Read the model definition and answer for the solid it produces. Units are mm, in the model's axes. A direction names the side the tool comes from. Coordinates: 2 decimals unless noted, no trailing zeros. Order: outer loops, then holes, each group sorted by start corner. A loop starts at its lowest first (then second) coordinate and runs counter-clockwise, first axis right, second up. Notation, with made-up numbers: (14, 3.25) -> (19, 3.25) arc R12 ccw to (19, 19.25) -> close; hole circle Ø4 at (64, 66.5). An arc over 180 degrees is marked (long way). Use CSV: the item, a comma, the result in double quotes.
```python
from build123d import *

# Parameters (mm, degrees)
F1_DEPTH = 7.14375
F2_W     = 15.875
F2_H     = 14.2875
F3_DEPTH = 9.525


with BuildPart() as f1:
    # F0 (on Top) → F1 (new body, symmetric)
    with BuildSketch(Plane.XY):
        Polygon((40.48125, 53.975), (40.48125, 9.525), (-40.48125, 9.525), (-40.48125, 53.975), (-53.18125, 53.975), (-53.18125, 9.525), (-53.18125, -9.525), (-40.48125, -9.525), (40.48125, -9.525), (53.18125, -9.525), (53.18125, 9.525), (53.18125, 53.975), align=None)
    extrude(amount=F1_DEPTH, both=True)

    # F2 (on face) → F3 (join)
    with BuildSketch(Plane(origin=(-53.18125, 0, 0), x_dir=(0, -1, 0), z_dir=(-1, 0, 0))):
        with Locations((-38.1, 0)):
            Rectangle(F2_W, F2_H)
    extrude(amount=F3_DEPTH)


solid = f1.part
```
Item 1: Find section A-A, the plane y = 19. Give the vertices of the cut face in (x, z).
Return value:
outline,"(-53.18, -7.14) -> (-40.48, -7.14) -> (-40.48, 7.14) -> (-53.18, 7.14) -> close; (40.48, -7.14) -> (53.18, -7.14) -> (53.18, 7.14) -> (40.48, 7.14) -> close"
Item 2: Straight lines are drawn through the part: line 1 along X through (y, z) = (43.5, -2.25); line 2 along X through (y, z) = (12.5, 1.25); line 3 along X through (y, z) = (-6.5, 0.75). For each, find the intervals that lie inside material, in ascending order.
Return value:
line 1,"x = -62.71 to -40.48, 40.48 to 53.18"
line 2,"x = -53.18 to -40.48, 40.48 to 53.18"
line 3,"x = -53.18 to 53.18"
Item 3: The mould has two halves that part along X. Classify faces 1 (the flat face through (-6, 9, -7.144)), 2 (the flat face through (1, 9.525, 0)), 3 (the flat face through (-40.481, 31, 0)), 4 (the flat face through (53.181, 22, 0)): +X half, -X half, draft (parallel to the pull), parting line (faces both ways), or undercut.
Return value:
face 1,"draft"
face 2,"undercut"
face 3,"undercut"
face 4,"+X half"
Item 4: A tool of negligible diameter and unlimited length cuts with its end or side. For faces 5 (the flat face through (-58, 30.162, 0)), 6 (the flat face through (40.481, 32, 0)), 7 (the flat face through (-6, 9, 7.144)), 8 (the flat face through (-53.181, 50, 0)), from which of +Z, -Z, +X, -X, +Y, -Y can it reach the whole face along a straight path? Write none if from no direction.
Return value:
face 5,"+Z, -Z, -X, -Y"
face 6,"+Z, -Z, +Y"
face 7,"+Z, +X, -X, +Y, -Y"
face 8,"+Z, -Z, -X, +Y"
Item 5: Find section C-C, the plane y = 33.5. Give the vertices of the cut face in (x, z).
Return value:
outline,"(-62.71, -7.14) -> (-40.48, -7.14) -> (-40.48, 7.14) -> (-62.71, 7.14) -> close; (40.48, -7.14) -> (53.18, -7.14) -> (53.18, 7.14) -> (40.48, 7.14) -> close"
Item 6: Each of these flat-tipped pins is pushed along its axis until it touches: P1, Ø4, axis at y = 6.5, z = 3.5, coming from the -X side; P2, Ø7.5, axis at x = -57, z = 1, coming from the +Y side; P3, Ø4.5, axis at x = -0.5, z = -1, coming from the +Y side (3 decimals). Where does it stop, or does it pass through?
Return value:
P1,"stops at x = -53.18"
P2,"stops at y = 46.04"
P3,"stops at y = 9.525"
Item 7: Find section B-B, the plane z = 5. Give the vertices of the cut face in (x, y) (1 decimal), then the cut area to 3 significant figures.
Return value:
outline,"(-62.7, 30.2) -> (-53.2, 30.2) -> (-53.2, -9.5) -> (53.2, -9.5) -> (53.2, 54) -> (40.5, 54) -> (40.5, 9.5) -> (-40.5, 9.5) -> (-40.5, 54) -> (-53.2, 54) -> (-53.2, 46) -> (-62.7, 46) -> close"
area,"3,310 mm^2"
Item 8: Find section D-D, the plane x = -19.5. Give the vertices of the cut face in (y, z) (3 decimals).
Return value:
outline,"(-9.525, -7.144) -> (9.525, -7.144) -> (9.525, 7.144) -> (-9.525, 7.144) -> close"
